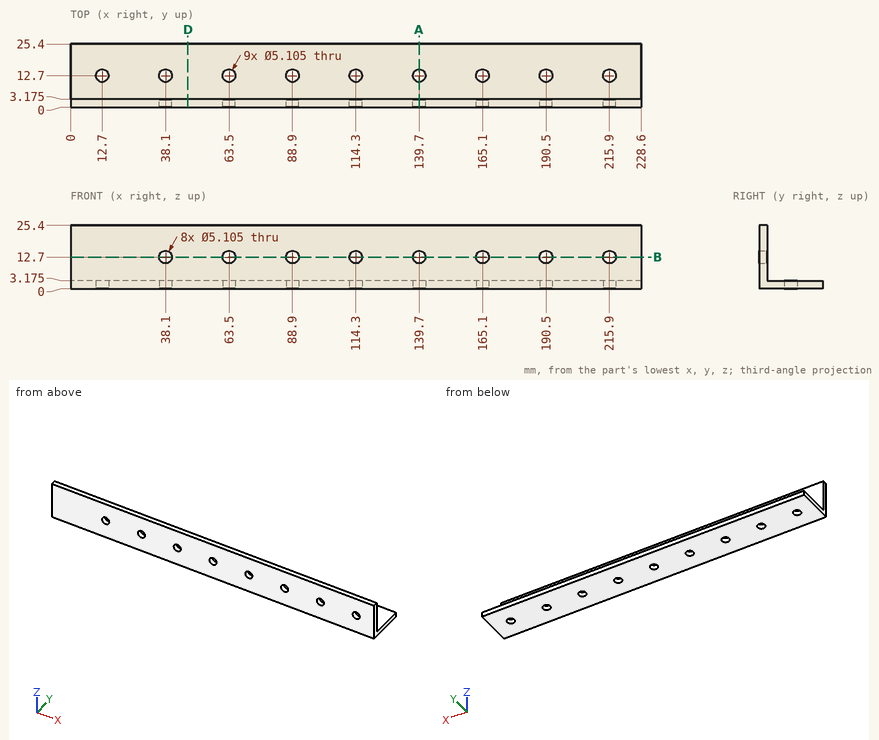
Could you check a few things on this drawing? It's one solid part, dimensions in mm from its lowest x, y, z. Give positions to 0.01 mm unless a question says otherwise; leave off trailing zeros. Loops run counter-clockwise (first coordinate to the right, second up) from the corner with the lowest first, then second, coordinate; pieces in that order, holes last. Notation, with made-up numbers: M -17,-6.5 L 37,-6.5 A5 cw 37,1.5 Z; hole C 39,5.25 d7. An arc over 180 degrees is marked long. One line per question, with ' | ' between items. Start each with the question number.
Q1. For pin 1 Ø4.5 at (x, z) = (165.1, 12.7) entering from -Y; pin 2 Ø6.5 at (x, y) = (142, 19) entering from +Z (3 decimals); pin 3 Ø8 at (x, z) = (63.5, 12.7) entering from +Y (3 decimals), each with a flat end and sliding along its axis, tell me the tip position at first contact or that it passes through.
Q2. If I drill on line 1 (Z direction, x = 215.9, y = 2.4); line 2 (Y direction, x = 83, z = 24) (1 decimal), over which ranges is the centre line in solid material (lowest first)? Write a range as from..to.
Q3. If we section it at D-D (x = 47): Please give me the cut outline in (y, z) (1 decimal).
Q4. If we section it at B-B (z = 12.7): State how many separate pieces and enclosed holes the cut face has, plus the area to 3 significant figures.
Q5. If we section it at A-A (x = 139.7): Please give me the cut outline in (y, z) (1 decimal).
Computed:
1) pin 1: passes through | pin 2: stops at z = 3.175 | pin 3: stops at y = 3.175
2) line 1: z = 0..10.15, 15.25..25.4 | line 2: y = 0..3.2
3) outline: M 0,0 L 25.4,0 L 25.4,3.2 L 3.2,3.2 L 3.2,25.4 L 0,25.4 Z
4) separate pieces: 9 | enclosed holes: 0 | area: 596 mm²
5) outline: M 0,0 L 10.1,0 L 10.1,3.2 L 3.2,3.2 L 3.2,10.1 L 0,10.1 Z; M 0,15.3 L 3.2,15.3 L 3.2,25.4 L 0,25.4 Z; M 15.3,0 L 25.4,0 L 25.4,3.2 L 15.3,3.2 Z
